Build history of the part. All positions in model axes, mm. A direction names the side the tool comes from. Coordinates: 2 decimals unless noted, no trailing zeros. Loops run counter-clockwise (first coordinate to the right, second up) from the corner with the lowest first, then second, coordinate; pieces in that order, holes last. Notation, with made-up numbers: (-14.5, 18.5) - (4.5, 18.5) arc R23 ccw to (4.5, 32.5) - close; hole circle Ø3 at (69.25, -37). An arc over 180 degrees is marked (long way). One line per item, written item: value.
```python
from build123d import *

# Parameters (mm, degrees)
F1_DEPTH = 10
F2_D     = 8
F2_DEPTH = 25
F2_TIP   = 2.4034424761
F3_D     = 10.4
F3_DEPTH = 4.3
F3_TIP   = 3.1244752189


with BuildPart() as f1:
    # F0 (on Front) → F1 (new body)
    with BuildSketch(Plane.XZ):
        with BuildLine():
            Line((-75, 10), (-75, 0))
            Line((-75, 0), (75, 0))
            Line((75, 0), (75, 10))
            Line((75, 10), (6.4358378053, 67.6537567079))
            ThreePointArc((6.4358378053, 67.6537567079), (0, 70), (-6.4358378053, 67.6537567079))
            Line((-6.4358378053, 67.6537567079), (-75, 10))
        make_face()
        Polygon((-13.1993114793, 10), (-59.46200743, 10), (-37.3569899514, 28.587513636), align=None, mode=Mode.SUBTRACT)
        with BuildLine():
            Line((-29.5214792948, 35.1761834399), (-7.6537567079, 53.5641621947))
            ThreePointArc((-7.6537567079, 53.5641621947), (-6.4238926361, 52.3362148125), (-5, 51.3397459622))
            Line((-5, 51.3397459622), (-5, 16.3087524782))
            Line((-5, 16.3087524782), (-29.5214792948, 35.1761834399))
        make_face(mode=Mode.SUBTRACT)
        Polygon((37.3569899514, 28.587513636), (59.46200743, 10), (13.1993114793, 10), align=None, mode=Mode.SUBTRACT)
        with BuildLine():
            ThreePointArc((5, 51.3397459622), (6.4238926361, 52.3362148125), (7.6537567079, 53.5641621947))
            Line((7.6537567079, 53.5641621947), (29.5214792948, 35.1761834399))
            Line((29.5214792948, 35.1761834399), (5, 16.3087524782))
            Line((5, 16.3087524782), (5, 51.3397459622))
        make_face(mode=Mode.SUBTRACT)
    extrude(amount=F1_DEPTH)

    # F2
    with Locations(Plane(origin=(0, 0, 0), x_dir=(1, 0, 0), z_dir=(0, 1, 0))):
        with Locations((0, -60)):
            Hole(F2_D / 2, depth=F2_DEPTH)
            with Locations((0, 0, -(F2_DEPTH + F2_TIP / 2))):  # 118° drill point
                Cone(0, F2_D / 2, F2_TIP, mode=Mode.SUBTRACT)

    # F3
    with Locations(Plane(origin=(0, 0, 0), x_dir=(1, 0, 0), z_dir=(0, 1, 0))):
        with Locations((0, -60)):
            Hole(F3_D / 2, depth=F3_DEPTH)
            with Locations((0, 0, -(F3_DEPTH + F3_TIP / 2))):  # 118° drill point
                Cone(0, F3_D / 2, F3_TIP, mode=Mode.SUBTRACT)


solid = f1.part
```
Item 1: Drop flat-ended pins along their axis: P1, Ø6, axis at x = 0, z = 60, coming from the -Y side; P2, Ø6, axis at y = -8, z = 35, coming from the -X side; P3, Ø4, axis at y = -5, z = 47, coming from the -X side; P4, Ø5, axis at x = 29.5, y = -3, coming from the +Z side. Give the stop position or say it passes through.
Check result:
P1: passes through
P2: stops at x = -48.84
P3: stops at x = -33.38
P4: stops at z = 50.36
Item 2: Cut at C-C, the plane z = 60. Write the cut outline in (x, y), then the cut area to 3 significant figures.
Check result:
outline: (-15.54, -10) - (-4, -10) - (-4, -5.02) - (-5.2, -4.3) - (-5.2, 0) - (-15.54, 0) - close; (4, -10) - (15.54, -10) - (15.54, 0) - (5.2, 0) - (5.2, -4.3) - (4, -5.02) - close
area: 220 mm^2
Item 3: Tool access for faces 1 (the face through (41.2, -4.93, 38.42)), 2 (the face through (17.432, -4.93, 25.875)): list every direction of +Z, -Z, +X, -X, +Y, -Y with a clear straight run to the whole face (end or side of a thin tool).
Check result:
face 1: +Z, +X, +Y, -Y
face 2: +Y, -Y
Item 4: Cut at A-A, the plane y = -2. Write the cut outline in (x, z), then the cut area to 3 significant figures.
Check result:
outline: (-75, 0) - (75, 0) - (75, 10) - (6.44, 67.65) arc R10 ccw to (-6.44, 67.65) - (-75, 10) - close; hole (-59.46, 10) - (-13.2, 10) - (-37.36, 28.59) - close; hole (-29.52, 35.18) - (-5, 16.31) - (-5, 51.34) arc R10 cw to (-7.65, 53.56) - close; hole circle Ø10.4 at (0, 60); hole (5, 16.31) - (29.52, 35.18) - (7.65, 53.56) arc R10 cw to (5, 51.34) - close; hole (13.2, 10) - (59.46, 10) - (37.36, 28.59) - close
area: 4,320 mm^2
Item 5: Pull direction Z, two halves, no side cores. Call faces 3 (the face through (-40.24, -4.93, 39.23)), 4 (the face through (-1, -10, 28)), 5 (the face through (0.677, -2.18, 54.844)), 6 (the face through (-1, -5, 0)): released by +Z, released by -Z, zero draft, split by the parting line, or undercut.
Check result:
face 3: released by +Z
face 4: zero draft
face 5: undercut
face 6: released by -Z
Item 6: Cut at B-B, the plane x = 0. Write the cut outline in (y, z).
Check result:
outline: (-10, 0) - (0, 0) - (0, 54.8) - (-4.3, 54.8) - (-5.02, 56) - (-10, 56) - close; (-10, 64) - (-5.02, 64) - (-4.3, 65.2) - (0, 65.2) - (0, 70) - (-10, 70) - close
Item 7: Probe probe 1 along X at (y, z) = (-8.5, 44.5); probe 2 along X at (y, z) = (-8.25, 37); probe 3 along Z at (x, y) = (0, -2.2). List the from-to ranges inside material, lowest first. Write a range as from..to.
Check result:
probe 1: x = -33.97..-18.43, -5..5, 18.43..33.97
probe 2: x = -42.89..-27.35, -5..5, 27.35..42.89
probe 3: z = 0..54.8, 65.2..70
Item 8: Cut at D-D, the plane x = 23. Write the cut outline in (y, z).
Check result:
outline: (-10, 0) - (0, 0) - (0, 10) - (-10, 10) - close; (-10, 17.54) - (0, 17.54) - (0, 30.16) - (-10, 30.16) - close; (-10, 40.66) - (0, 40.66) - (0, 53.73) - (-10, 53.73) - close
